```python
from build123d import *

# Parameters (mm, degrees)
SKETCH1_R           = 4.445
BOSS_EXTRUDE1_DEPTH = 3.81
FILLET2_R           = 1.27
SKETCH2_R           = 2.54
BOSS_EXTRUDE2_DEPTH = 35.56


with BuildPart() as part:
    # Sketch1 → Boss-Extrude1 (new body)
    with BuildSketch(Plane.XY):
        with Locations(Location((0, 0, 0), (0, 0, 180))):
            Circle(SKETCH1_R)
    extrude(amount=BOSS_EXTRUDE1_DEPTH)

    # Fillet2
    fillet2_edges = [part.edges().sort_by_distance(p)[0] for p in [
        (4.445, 0, 3.81),
    ]]
    fillet(fillet2_edges, radius=FILLET2_R)

    # Sketch2 → Boss-Extrude2 (add)
    with BuildSketch(Plane(origin=(0, 0, 0), x_dir=(-1, 0, 0), z_dir=(0, 0, -1))):
        with Locations(Location((0, 0, 0), (0, 0, 180))):
            Circle(SKETCH2_R)
    extrude(amount=BOSS_EXTRUDE2_DEPTH)


solid = part.part
```
Work out the finished part from the listing and answer in its coordinate system (mm). Give positions to 0.01 mm unless a question says otherwise; leave off trailing zeros. Write each loop counter-clockwise with the first axis right and the second up, starting at its lowest first coordinate (ties: lowest second). Pieces come first, ordered by that corner, then holes.
(1) Flat-ended cylindrical pins translate along their axes: pin 1 Ø4 at (y, z) = (-3.5, -25) entering from +X; pin 2 Ø1.5 at (x, z) = (-1, -20) entering from +Y; pin 3 Ø2 at (y, z) = (0.5, -2) entering from +X. Find the tip coordinate at first contact, or state that the pin passes through.
Final values:
pin 1: stops at x = 2.05
pin 2: stops at y = 2.53
pin 3: stops at x = 2.54
(2) The part is cut by section C-C on z = -29.5. Write down the section's boundary in (x, y), plus the area to 3 significant figures.
Final values:
outline: circle Ø5.08 at (0, 0)
area: 20.3 mm2
(3) The mould has two halves that part along Y. Classify faces 1 (the cylindrical face through (-0.33, -2.52, -17.53)), 2 (the flat face through (-2, 2, 0)): pulls with the +Y half, pulls with the -Y half, needs draft (parallel to the pull), parting line crosses it, or undercut.
Final values:
face 1: parting line crosses it
face 2: needs draft
(4) Straight lines are drawn through the part: line 1 (Z direction, x = -2.5, y = -0.75); line 2 (X direction, y = 0.5, z = -5.5). For each, find the intervals that lie inside material, in ascending order.
Final values:
line 1: z = 0 to 3.81
line 2: x = -2.49 to 2.49
(5) The part is cut by section A-A on x = 0. Write down the section's boundary in (y, z) (3 decimals), plus the area to 3 significant figures.
Final values:
outline: (-4.445, 0) - (-2.54, 0) - (-2.54, -35.56) - (2.54, -35.56) - (2.54, 0) - (4.445, 0) - (4.445, 2.54) arc R1.27 ccw to (3.175, 3.81) - (-3.175, 3.81) arc R1.27 ccw to (-4.445, 2.54) - close
area: 214 mm2
